Print and shaded views of the part. All mm, measured from the part's lowest x, y and z. Round coordinates to 2 decimals unless told otherwise and drop trailing zeros. Loops run counter-clockwise (first coordinate to the right, second up) from the corner with the lowest first, then second, coordinate; pieces in that order, holes last. Notation, with made-up numbers: (-11.5, 59.5) -> (25.5, 59.5) arc R22 ccw to (25.5, 88.5) -> close; hole circle Ø5 at (-5.75, 58). An arc over 180 degrees is marked (long way). Answer as CSV lines item,"result".
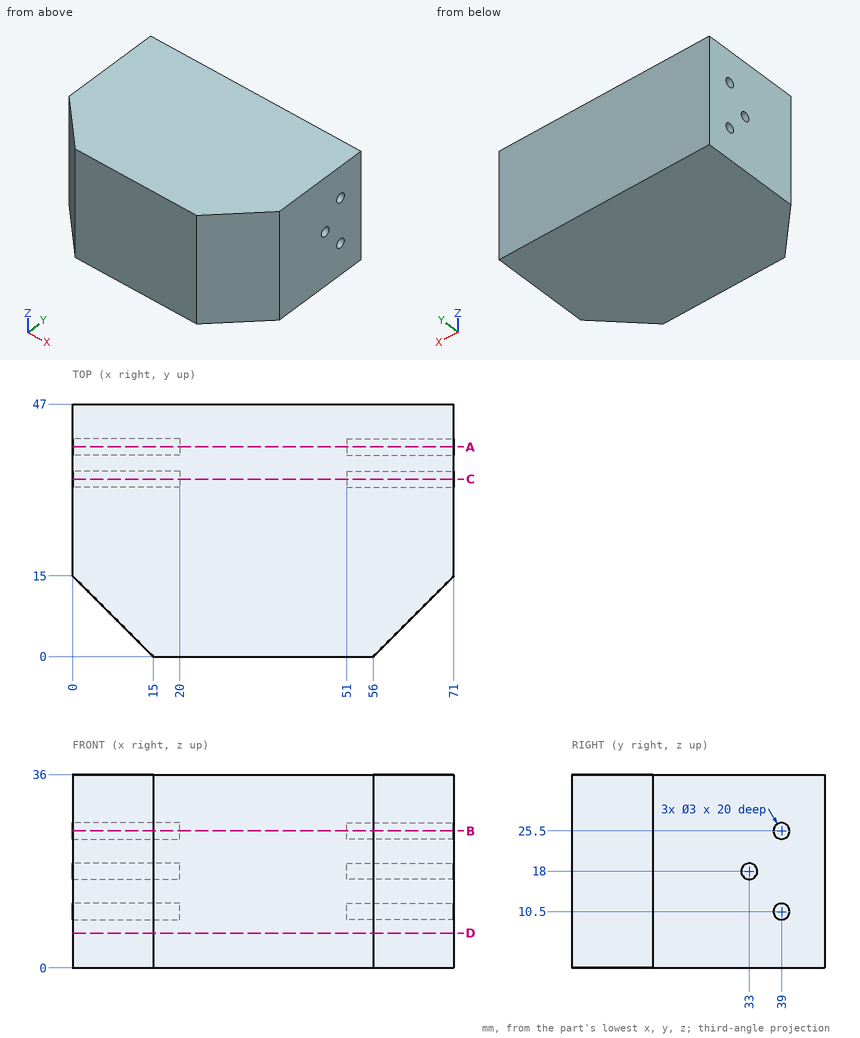
Q1. Slice it at A-A, the plane y = 39. Give the cut face in (x, z).
Results:
outline,"(0, 0) -> (71, 0) -> (71, 9) -> (51, 9) -> (51, 12) -> (71, 12) -> (71, 24) -> (51, 24) -> (51, 27) -> (71, 27) -> (71, 36) -> (0, 36) -> (0, 27) -> (20, 27) -> (20, 24) -> (0, 24) -> (0, 12) -> (20, 12) -> (20, 9) -> (0, 9) -> close"
Q2. Slice it at D-D, the plane z = 6.5. Give the cut face in (x, y).
Results:
outline,"(0, 15) -> (15, 0) -> (56, 0) -> (71, 15) -> (71, 47) -> (0, 47) -> close"
Q3. Slice it at B-B, the plane z = 25.5. Give the cut face in (x, y), and give its area (3 significant figures).
Results:
outline,"(0, 15) -> (15, 0) -> (56, 0) -> (71, 15) -> (71, 37.5) -> (51, 37.5) -> (51, 40.5) -> (71, 40.5) -> (71, 47) -> (0, 47) -> (0, 40.5) -> (20, 40.5) -> (20, 37.5) -> (0, 37.5) -> close"
area,"2,990 mm2"
Q4. Drop flat-ended pins along their axis: pin 1 Ø2.5 at (y, z) = (39, 10.5) entering from -X; pin 2 Ø1.8 at (y, z) = (39, 10.5) entering from +X; pin 3 Ø4 at (y, z) = (10, 12) entering from -X. Give the stop position or say it passes through.
Results:
pin 1,"x = 20"
pin 2,"x = 51"
pin 3,"x = 3"
Q5. Slice it at C-C, the plane y = 33. Give the cut face in (x, z).
Results:
outline,"(0, 0) -> (71, 0) -> (71, 16.5) -> (51, 16.5) -> (51, 19.5) -> (71, 19.5) -> (71, 36) -> (0, 36) -> (0, 19.5) -> (20, 19.5) -> (20, 16.5) -> (0, 16.5) -> close"
Q6. Probe L1, parallel to Y at x = 63.75, z = 18; L2, parallel to Y at x = 59, z = 10.5; L3, parallel to X at y = 33, z = 19. List the from-to ranges inside material, lowest first. Write a range as [from, to].
Results:
L1,"[7.75, 31.5], [34.5, 47]"
L2,"[3, 37.5], [40.5, 47]"
L3,"[20, 51]"
